```python
from build123d import *

# Parameters (mm, degrees)
ESQUISSE1_W             = 15
ESQUISSE1_H             = 15
EXTRUSION1_DEPTH        = 100
ESQUISSE2_W             = 12
ESQUISSE2_H             = 12
EXTRUSION2_DEPTH        = 101.560926806
CONG_1_R                = 7.5
ESQUISSE3_R             = 1.5
EXTRUSION3_DEPTH        = 102.396498953
ESQUISSE4_W             = 12
ESQUISSE4_H             = 14
ENL_V_MAT_EXTRU_1_DEPTH = 3


with BuildPart() as part:
    # Esquisse1 → Extrusion1 (new body)
    with BuildSketch(Plane.XY):
        Rectangle(ESQUISSE1_W, ESQUISSE1_H)
    extrude(amount=EXTRUSION1_DEPTH)

    # Esquisse2 → Extrusion2 (cut, through all)
    with BuildSketch(Plane.XY.offset(100)):
        Rectangle(ESQUISSE2_W, ESQUISSE2_H)
    extrude(amount=-EXTRUSION2_DEPTH, mode=Mode.SUBTRACT)

    # Congé1
    # the kernel refuses this fillet: 7.5 mm, written as the material it takes off along each edge
    with BuildSketch(Plane(origin=(-26.25, -7.5, 0), x_dir=(0, 0, 1), z_dir=(1, 0, 0))) as cong_1_piece_1:
        with BuildLine():
            CenterArc((CONG_1_R, -CONG_1_R), CONG_1_R, 90, 90)
            Line((0, -CONG_1_R), (0, 0))
            Line((0, 0), (CONG_1_R, 0))
        make_face()
    extrude(amount=52.5, mode=Mode.SUBTRACT)
    with BuildSketch(Plane(origin=(26.25, 7.5, 0), x_dir=(0, -1, 0), z_dir=(-1, 0, 0))) as cong_1_piece_2:
        with BuildLine():
            CenterArc((CONG_1_R, CONG_1_R), CONG_1_R, 180, 90)
            Line((0, CONG_1_R), (0, 0))
            Line((0, 0), (CONG_1_R, 0))
        make_face()
    extrude(amount=52.5, mode=Mode.SUBTRACT)

    # Esquisse3 → Extrusion3 (cut, through all)
    with BuildSketch(Plane(origin=(7.5, 0, 0), x_dir=(0, 0, -1), z_dir=(1, 0, 0))):
        with Locations((-7.5, 0)):
            Circle(ESQUISSE3_R)
    extrude(amount=-EXTRUSION3_DEPTH, mode=Mode.SUBTRACT)

    # Esquisse4 → Enlèv. mat.-Extru.1 (cut)
    with BuildSketch(Plane(origin=(0, 7.5, 0), x_dir=(-1, 0, 0), z_dir=(0, 1, 0))):
        with Locations((0, 32.5)):
            Rectangle(ESQUISSE4_W, ESQUISSE4_H)
    extrude(amount=-ENL_V_MAT_EXTRU_1_DEPTH, mode=Mode.SUBTRACT)


solid = part.part
```
For this review, take the finished solid that the model builds, in its own axes (mm). A direction names the side the tool comes from. Coordinates: 2 decimals unless noted, no trailing zeros. Write each loop counter-clockwise with the first axis right and the second up, starting at its lowest first coordinate (ties: lowest second). Pieces come first, ordered by that corner, then holes. Notation, with made-up numbers: (70, 89.25) -> (117, 89.25) arc R27 ccw to (117, 123.25) -> close; hole circle Ø9 at (16.5, -5). An arc over 180 degrees is marked (long way). Put each result on its own line as item: value.
Q1. The part is to be moulded in two halves that separate along Y. For faces 3 (the flat face through (7.5, 0, 49)), 4 (the cylindrical face through (0.105, 6.576, 3.894)), 5 (the cylindrical face through (7, 0, 9)), say which applies: +Y half, -Y half, draft (parallel to the pull), parting line (faces both ways), or undercut.
From the geometry:
face 3: draft
face 4: parting line
face 5: undercut
Q2. Wall thickness on L1, parallel to Y at x = 1, z = 52; L2, parallel to Y at x = -6.45, z = 7.5: over which ranges is each line inside the solid? List them lowest first.
From the geometry:
L1: y = -7.5 to -6, 6 to 7.5
L2: y = -7.5 to -1.5, 1.5 to 7.5
Q3. Tool access review of faces 1 (the flat face through (0, -7.5, 53)), 2 (the flat face through (0, 6, 14)): name each direction out of +Z, -Z, +X, -X, +Y, -Y from which nothing blocks a thin tool from reaching the whole face with its end or side.
From the geometry:
face 1: +Z, -Z, +X, -X, -Y
face 2: +Z, -Z
Q4. Clearance check with flat-ended pins moving along their axes: pin 1 Ø2.5 at (y, z) = (0, 7.5) entering from +X; pin 2 Ø1.6 at (x, y) = (2.5, 6.5) entering from -Z. State where each tip first meets the part, or that it passes through.
From the geometry:
pin 1: passes through
pin 2: stops at z = 3
Q5. Take a section at B-B, the plane y = 0. State the section outline as (x, z) points, then the cut area to 3 significant figures.
From the geometry:
outline: (-7.5, 0) -> (-6, 0) -> (-6, 6) -> (-7.5, 6) -> close; (-7.5, 9) -> (-6, 9) -> (-6, 100) -> (-7.5, 100) -> close; (6, 0) -> (7.5, 0) -> (7.5, 6) -> (6, 6) -> close; (6, 9) -> (7.5, 9) -> (7.5, 100) -> (6, 100) -> close
area: 291 mm2
Q6. Take a section at D-D, the plane z = 27.5. State the section outline as (x, y) points, then the cut area to 3 significant figures.
From the geometry:
outline: (-7.5, -7.5) -> (7.5, -7.5) -> (7.5, 7.5) -> (6, 7.5) -> (6, -6) -> (-6, -6) -> (-6, 7.5) -> (-7.5, 7.5) -> close
area: 63.0 mm2
Q7. Take a section at C-C, the plane z = 87.5. State the section outline as (x, y) points, then the cut area to 3 significant figures.
From the geometry:
outline: (-7.5, -7.5) -> (7.5, -7.5) -> (7.5, 7.5) -> (-7.5, 7.5) -> close; hole (-6, -6) -> (6, -6) -> (6, 6) -> (-6, 6) -> close
area: 81.0 mm2
Q8. Take a section at A-A, the plane x = -2.5. State the section outline as (y, z) points.
From the geometry:
outline: (-7.5, 7.5) arc R7.5 ccw to (-6, 3) -> (-6, 100) -> (-7.5, 100) -> close; (6, 3) arc R7.5 ccw to (7.5, 7.5) -> (7.5, 25.5) -> (6, 25.5) -> close; (6, 39.5) -> (7.5, 39.5) -> (7.5, 100) -> (6, 100) -> close
